Model file for the job. Use its own axes, mm. Face numbers are marked on the shaded views. Round coordinates to 2 decimals unless told otherwise and drop trailing zeros. Write each loop counter-clockwise with the first axis right and the second up, starting at its lowest first coordinate (ties: lowest second). Pieces come first, ordered by that corner, then holes. Notation, with made-up numbers: (72.5, 85) - (104.5, 85) arc R6 cw to (104.5, 91) - close; hole circle Ø9 at (-34.5, -15). An arc over 180 degrees is marked (long way). One line per item, written item: value.
from build123d import *

# Parameters (mm, degrees)
SKETCH_1_W      = 66.19
SKETCH_1_H      = 27.25
EXTRUDE_1_DEPTH = 3


with BuildPart() as part:
    # 草图1 → 凸台-拉伸1 (new body)
    with BuildSketch(Plane(origin=(0, 0, 0), x_dir=(1, 0, 0), z_dir=(0, 1, 0))):
        Rectangle(SKETCH_1_W, SKETCH_1_H)
        with BuildLine():
            Line((-28.41294438, 12.875), (-23.41294438, 12.875))
            ThreePointArc((-23.41294438, 12.875), (-20.41294438, 9.875), (-23.41294438, 6.875))
            Line((-23.41294438, 6.875), (-28.41294438, 6.875))
            ThreePointArc((-28.41294438, 6.875), (-31.41294438, 9.875), (-28.41294438, 12.875))
        make_face(mode=Mode.SUBTRACT)
        with BuildLine():
            Line((28.41294438, 12.875), (23.41294438, 12.875))
            ThreePointArc((23.41294438, 12.875), (20.41294438, 9.875), (23.41294438, 6.875))
            Line((23.41294438, 6.875), (28.41294438, 6.875))
            ThreePointArc((28.41294438, 6.875), (31.41294438, 9.875), (28.41294438, 12.875))
        make_face(mode=Mode.SUBTRACT)
        with BuildLine():
            Line((-28.41294438, -12.875), (-23.41294438, -12.875))
            ThreePointArc((-23.41294438, -12.875), (-20.41294438, -9.875), (-23.41294438, -6.875))
            Line((-23.41294438, -6.875), (-28.41294438, -6.875))
            ThreePointArc((-28.41294438, -6.875), (-31.41294438, -9.875), (-28.41294438, -12.875))
        make_face(mode=Mode.SUBTRACT)
        with BuildLine():
            Line((28.41294438, -12.875), (23.41294438, -12.875))
            ThreePointArc((23.41294438, -12.875), (20.41294438, -9.875), (23.41294438, -6.875))
            Line((23.41294438, -6.875), (28.41294438, -6.875))
            ThreePointArc((28.41294438, -6.875), (31.41294438, -9.875), (28.41294438, -12.875))
        make_face(mode=Mode.SUBTRACT)
    extrude(amount=EXTRUDE_1_DEPTH)


solid = part.part
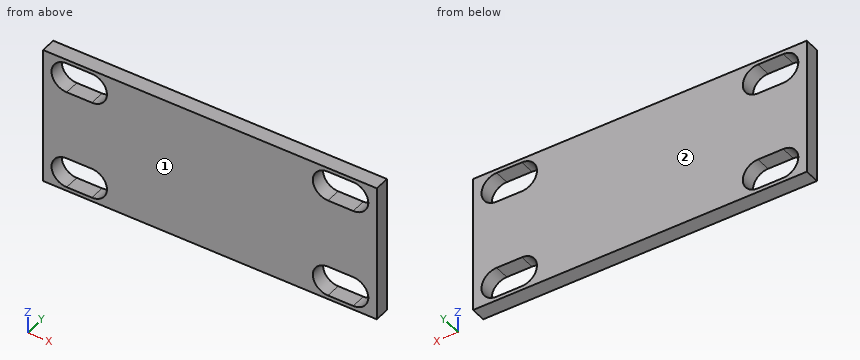
1. Band-saw the part on C-C on y = 1.15. Write the cut outline in (x, z) (3 decimals).
Report:
outline: (-33.095, -13.625) - (33.095, -13.625) - (33.095, 13.625) - (-33.095, 13.625) - close; hole (-28.413, -12.875) - (-23.413, -12.875) arc R3 ccw to (-23.413, -6.875) - (-28.413, -6.875) arc R3 ccw to start; hole (-28.413, 6.875) - (-23.413, 6.875) arc R3 ccw to (-23.413, 12.875) - (-28.413, 12.875) arc R3 ccw to start; hole (23.413, -12.875) - (28.413, -12.875) arc R3 ccw to (28.413, -6.875) - (23.413, -6.875) arc R3 ccw to start; hole (23.413, 6.875) - (28.413, 6.875) arc R3 ccw to (28.413, 12.875) - (23.413, 12.875) arc R3 ccw to start
2. Band-saw the part on A-A on x = 25. Write the cut outline in (y, z) (3 decimals).
Report:
outline: (0, -13.625) - (3, -13.625) - (3, -12.875) - (0, -12.875) - close; (0, -6.875) - (3, -6.875) - (3, 6.875) - (0, 6.875) - close; (0, 12.875) - (3, 12.875) - (3, 13.625) - (0, 13.625) - close
3. Mould opens along Y. For the marked faces 1 and 2 say: released by +Y, released by -Y, zero draft, split by the parting line, or undercut.
Report:
face 1: released by -Y
face 2: released by +Y
4. Wall check: probe 1 along Z at (x, y) = (-25.5, 0.25) (3 decimals); probe 2 along Z at (x, y) = (21, 1.9) (3 decimals); probe 3 along X at (y, z) = (1.25, 8.75) (3 decimals). Give the ranges that are in metal, low to high. Write a range as [from, to].
Report:
probe 1: [-13.625, -12.875], [-6.875, 6.875], [12.875, 13.625]
probe 2: [-13.625, -11.658], [-8.092, 8.092], [11.658, 13.625]
probe 3: [-33.095, -31.194], [-20.632, 20.632], [31.194, 33.095]
5. Band-saw the part on B-B on z = 7.5. Write the cut outline in (x, y) (3 decimals), plus the area to 3 significant figures.
Report:
outline: (-33.095, 0) - (-30.246, 0) - (-30.246, 3) - (-33.095, 3) - close; (-21.58, 0) - (21.58, 0) - (21.58, 3) - (-21.58, 3) - close; (30.246, 0) - (33.095, 0) - (33.095, 3) - (30.246, 3) - close
area: 147 mm²
6. Drop a flat-ended pin along its axis: pin 1 (5 mm diameter, centred on x = 23.5, z = -0.5, fed in from -Y). Give the stop position or say it passes through.
Report:
pin 1: y = 0
